from build123d import *

# Parameters (mm, degrees)
BOSS_EXTRUDE2_DEPTH = 60
FILLET3_R           = 10


with BuildPart() as part:
    # Sketch1 → Boss-Extrude2 (new body)
    with BuildSketch(Plane(origin=(0, 0, 0), x_dir=(1, 0, 0), z_dir=(0, 1, 0))):
        with BuildLine():
            Line((-65, 10.711576414), (-42.160551831, 10.711576414))
            ThreePointArc((-42.160551831, 10.711576414), (0, -43.5), (42.160551831, 10.711576414))
            Line((42.160551831, 10.711576414), (65, 10.711576414))
            Line((65, 10.711576414), (65, 16.568265676))
            Line((65, 16.568265676), (34.752590874, 16.568265676))
            ThreePointArc((34.752590874, 16.568265676), (0, -38.5), (-34.752590874, 16.568265676))
            Line((-34.752590874, 16.568265676), (-65, 16.568265676))
            Line((-65, 16.568265676), (-65, 10.711576414))
        make_face()
    extrude(amount=BOSS_EXTRUDE2_DEPTH)

    # Fillet3
    fillet3_edges = [part.edges().sort_by_distance(p)[0] for p in [
        (42.160551831, 30, -10.711576414),
        (-42.160551831, 30, -10.711576414),
    ]]
    fillet(fillet3_edges, radius=FILLET3_R)


solid = part.part
Check sheet for the modelled part. Datum: model origin and axes. Units: mm. A direction names the side the tool comes from. Give positions to 0.01 mm unless a question says otherwise; leave off trailing zeros. Loops run counter-clockwise (first coordinate to the right, second up) from the corner with the lowest first, then second, coordinate; pieces in that order, holes last. Notation, with made-up numbers: M -10.75,82 L 6.25,82 A28 ccw 6.25,120 Z; hole C 69.5,68 d2. An arc over 180 degrees is marked long. Answer as a JSON object with one key per item and string values. Group by question number.
Q1. Cross-section at D-D on z = 15.5. Record the cut outline in (x, y), then the cut area to 3 significant figures.
Q2. Go/stop test with flat-tipped pins: P1, Ø12.5, axis at x = 56.5, y = 28.5, coming from the +Z side; P2, Ø3, axis at y = 51, z = 19, coming from the -X side; P3, Ø6, axis at x = -57.5, y = 34.5, coming from the +Z side. Record where each tip stops, or that it passes through.
Q3. Material ranges on line 1 along X through (y, z) = (40, 0); line 2 along X through (y, z) = (33, 24.5); line 3 along X through (y, z) = (8.5, 39.5), recorded low to high. Write a range as [from, to].
Q4. Cross-section at A-A on z = 30. Record the cut outline in (x, y).
Q5. Cross-section at C-C on x = 0. Record the cut outline in (y, z), then the cut area to 3 significant figures.
Q6. Release check for a two-part mould opening along Z. For faces 3 (the flat face through (-50, 30, -16.568)), 4 (the flat face through (-59, 30, -10.712)), 5 (the cylindrical face through (1.086, 29.58, 38.485)), 6 (the flat face through (65, 30, -14)) record: released by +Z, released by -Z, zero draft, split by the parting line, or undercut.
Q7. Access from +Z, -Z, +X, -X, +Y, -Y to the whole of each face (thin tool, end or side, straight path). Record for faces 1 (the flat face through (50, 30, -16.568)), 2 (the flat face through (59, 30, -10.712)).
Evaluation:
{
 "1": {"outline": "M -40.64,0 L -35.24,0 L -35.24,60 L -40.64,60 Z; M 35.24,0 L 40.64,0 L 40.64,60 L 35.24,60 Z", "area": "648 mm2"},
 "2": {"P1": "stops at z = -10.17", "P2": "stops at x = -39.82", "P3": "stops at z = -10.71"},
 "3": {"line 1": "x = [-43.5, -38.5], [38.5, 43.5]", "line 2": "x = [-35.94, -29.7], [29.7, 35.94]", "line 3": "x = [-18.22, 18.22]"},
 "4": {"outline": "M -31.5,0 L -24.13,0 L -24.13,60 L -31.5,60 Z; M 24.13,0 L 31.5,0 L 31.5,60 L 24.13,60 Z"},
 "5": {"outline": "M 0,38.5 L 60,38.5 L 60,43.5 L 0,43.5 Z", "area": "300 mm2"},
 "6": {"face 3": "released by -Z", "face 4": "released by +Z", "face 5": "undercut", "face 6": "zero draft"},
 "7": {"face 1": "-Z, +X, -X, +Y, -Y", "face 2": "+Z, +X, +Y, -Y"}
}
